```python
from build123d import *

# Parameters (mm, degrees)
F0_R     = 8
F1_DEPTH = 1
F3_DEPTH = 7
F4_R     = 8
F5_DEPTH = 1
F6_R     = 2.5
F7_DEPTH = 9


with BuildPart() as f1:
    # F0 (on Top) → F1 (new body)
    with BuildSketch(Plane.XY):
        Circle(F0_R)
    extrude(amount=F1_DEPTH)

    # F2 (on face) → F3 (join)
    with BuildSketch(Plane.XY.offset(1)):
        with BuildLine():
            Line((3.2969840058, 5.4029047423), (2.5065493984, 5.8119440209))
            ThreePointArc((2.5065493984, 5.8119440209), (1.8388116131, 5.5402736363), (1.4660287385, 6.1572918501))
            Line((1.4660287385, 6.1572918501), (0.587880666, 6.3020535948))
            ThreePointArc((0.587880666, 6.3020535948), (0.0367750598, 5.8373373817), (-0.5084316362, 6.3089603312))
            Line((-0.5084316362, 6.3089603312), (-1.3883339221, 6.1752742538))
            ThreePointArc((-1.3883339221, 6.1752742538), (-1.3836134942, 6.133709972), (-1.3820370329, 6.0919082168))
            ThreePointArc((-1.3820370329, 6.0919082168), (-1.8091754115, 5.5518374754), (-2.4331231799, 5.843063818))
            Line((-2.4331231799, 5.843063818), (-3.2286487127, 5.4440160432))
            ThreePointArc((-3.2286487127, 5.4440160432), (-3.1846641182, 5.3230332658), (-3.1697348597, 5.1951716444))
            ThreePointArc((-3.1697348597, 5.1951716444), (-3.5139617494, 4.6817520343), (-4.1196436741, 4.8052075072))
            Line((-4.1196436741, 4.8052075072), (-4.7529208721, 4.1798596116))
            ThreePointArc((-4.7529208721, 4.1798596116), (-4.6344100765, 4.0006685847), (-4.5928296865, 3.7898954745))
            ThreePointArc((-4.5928296865, 3.7898954745), (-4.859335021, 3.3157690905), (-5.4029047423, 3.2969840058))
            Line((-5.4029047423, 3.2969840058), (-5.8119440209, 2.5065493984))
            ThreePointArc((-5.8119440209, 2.5065493984), (-5.5928926927, 2.3021325953), (-5.5120190767, 2.0136379298))
            ThreePointArc((-5.5120190767, 2.0136379298), (-5.707906552, 1.590479337), (-6.1572918501, 1.4660287385))
            Line((-6.1572918501, 1.4660287385), (-6.3020535948, 0.587880666))
            ThreePointArc((-6.3020535948, 0.587880666), (-5.9691677754, 0.3993839994), (-5.8373263682, 0.0402714747))
            ThreePointArc((-5.8373263682, 0.0402714747), (-5.9714385265, -0.3214997579), (-6.3089603312, -0.5084316362))
            Line((-6.3089603312, -0.5084316362), (-6.1752742538, -1.3883339221))
            ThreePointArc((-6.1752742538, -1.3883339221), (-5.7301369842, -1.5161491913), (-5.5369082168, -1.9370370329))
            ThreePointArc((-5.5369082168, -1.9370370329), (-5.6196087137, -2.228512897), (-5.843063818, -2.4331231799))
            Line((-5.843063818, -2.4331231799), (-5.4440160432, -3.2286487127))
            ThreePointArc((-5.4440160432, -3.2286487127), (-4.9036957803, -3.2524353565), (-4.6401716444, -3.7247348597))
            ThreePointArc((-4.6401716444, -3.7247348597), (-4.683090061, -3.938738252), (-4.8052075072, -4.1196436741))
            Line((-4.8052075072, -4.1196436741), (-4.1798596116, -4.7529208721))
            ThreePointArc((-4.1798596116, -4.7529208721), (-3.5758920821, -4.6357481031), (-3.2348954745, -5.1478296865))
            ThreePointArc((-3.2348954745, -5.1478296865), (-3.2506409589, -5.2790911335), (-3.2969840058, -5.4029047423))
            Line((-3.2969840058, -5.4029047423), (-2.5065493984, -5.8119440209))
            ThreePointArc((-2.5065493984, -5.8119440209), (-1.8823764829, -5.5277645611), (-1.4586379298, -6.0670190767))
            ThreePointArc((-1.4586379298, -6.0670190767), (-1.4604887179, -6.1123064857), (-1.4660287385, -6.1572918501))
            Line((-1.4660287385, -6.1572918501), (-0.587880666, -6.3020535948))
            ThreePointArc((-0.587880666, -6.3020535948), (-0.0367750598, -5.8373373817), (0.5084316362, -6.3089603312))
            Line((0.5084316362, -6.3089603312), (1.3883339221, -6.1752742538))
            ThreePointArc((1.3883339221, -6.1752742538), (1.7688612926, -5.5630018732), (2.4331231799, -5.843063818))
            Line((2.4331231799, -5.843063818), (3.2286487127, -5.4440160432))
            ThreePointArc((3.2286487127, -5.4440160432), (3.4013491773, -4.7441209815), (4.1196436741, -4.8052075072))
            Line((4.1196436741, -4.8052075072), (4.7529208721, -4.1798596116))
            ThreePointArc((4.7529208721, -4.1798596116), (4.7008893059, -3.460852474), (5.4029047423, -3.2969840058))
            Line((5.4029047423, -3.2969840058), (5.8119440209, -2.5065493984))
            ThreePointArc((5.8119440209, -2.5065493984), (5.5402736363, -1.8388116131), (6.1572918501, -1.4660287385))
            Line((6.1572918501, -1.4660287385), (6.3020535948, -0.587880666))
            ThreePointArc((6.3020535948, -0.587880666), (5.8373373817, -0.0367750598), (6.3089603312, 0.5084316362))
            Line((6.3089603312, 0.5084316362), (6.1752742538, 1.3883339221))
            ThreePointArc((6.1752742538, 1.3883339221), (5.5630018732, 1.7688612926), (5.843063818, 2.4331231799))
            Line((5.843063818, 2.4331231799), (5.4440160432, 3.2286487127))
            ThreePointArc((5.4440160432, 3.2286487127), (4.7441209815, 3.4013491773), (4.8052075072, 4.1196436741))
            Line((4.8052075072, 4.1196436741), (4.1798596116, 4.7529208721))
            ThreePointArc((4.1798596116, 4.7529208721), (3.460852474, 4.7008893059), (3.2969840058, 5.4029047423))
        make_face()
    extrude(amount=F3_DEPTH)

    # F4 (on face) → F5 (join)
    with BuildSketch(Plane.XY.offset(8)):
        Circle(F4_R)
    extrude(amount=F5_DEPTH)

    # F6 (on face) → F7 (cut)
    with BuildSketch(Plane.XY.offset(9)):
        Circle(F6_R)
    extrude(amount=-F7_DEPTH, mode=Mode.SUBTRACT)


solid = f1.part
```
Model file for the job. Use its own axes, mm. A direction names the side the tool comes from. Coordinates: 2 decimals unless noted, no trailing zeros. Write each loop counter-clockwise with the first axis right and the second up, starting at its lowest first coordinate (ties: lowest second). Pieces come first, ordered by that corner, then holes. Notation, with made-up numbers: (-9.75, 39.5) - (48.25, 39.5) arc R19 cw to (48.25, 65.5) - close; hole circle Ø6 at (85.5, -14.75). An arc over 180 degrees is marked (long way). Use a Markdown table: item, result. Add a question column.
Item 1: Band-saw the part on A-A, the plane x = 0. Write the cut outline in (y, z), and give its area (3 significant figures).
Item 2: Two-plate mould, pull along Y, no slides. Class faces 1 (the face through (0.048, 5.837, 4.451)), 2 (the face through (-6.243, -0.942, 4.451)), 3 (the face through (5.837, -0.048, 4.451)): pulls with the +Y half, pulls with the -Y half, needs draft (parallel to the pull), parting line crosses it, or undercut.
Item 3: Drill centre lines: line 1 along Z through (x, y) = (2, 6.5); line 2 along Y through (x, z) = (0, 5.5); line 3 along X through (y, z) = (1.5, 0.75). Where is each one in solid material? Low to high.
Item 4: 3-axis set-ups, long thin cutter, end or side, ignore diameter. For faces 4 (the face through (-1.73, -7.81, 8.49)), 5 (the face through (-6.23, 1.03, 4.45)), 6 (the face through (3.47, 4.694, 4.451)), 7 (the face through (1.03, 6.23, 4.45)), 8 (the face through (0.942, -6.243, 4.451)): which of +Z, -Z, +X, -X, +Y, -Y reach the whole face in a straight line?
Item 5: Band-saw the part on B-B, the plane z = 8.5. Write the cut outline in (x, y), and give its area (3 significant figures).
Item 6: Drop flat-ended pins along their axis: pin 1 (4.5 mm diameter, centred on x = 0, y = 0, fed in from -Z); pin 2 (2 mm diameter, centred on x = 1, z = 2.5, fed in from +Y). Give the stop position or say it passes through.
A:
| question | item | result |
|---|---|---|
| 1 | outline | (-8, 0) - (-2.5, 0) - (-2.5, 9) - (-8, 9) - (-8, 8) - (-5.84, 8) - (-5.84, 1) - (-8, 1) - close; (2.5, 0) - (8, 0) - (8, 1) - (5.84, 1) - (5.84, 8) - (8, 8) - (8, 9) - (2.5, 9) - close |
| 1 | area | 68.7 mm² |
| 2 | face 1 | pulls with the +Y half |
| 2 | face 2 | pulls with the -Y half |
| 2 | face 3 | undercut |
| 3 | line 1 | z = 0 to 1, 8 to 9 |
| 3 | line 2 | y = -5.84 to -2.5, 2.5 to 5.84 |
| 3 | line 3 | x = -7.86 to -2, 2 to 7.86 |
| 4 | face 4 | +Z, -Z |
| 4 | face 5 | -X, +Y |
| 4 | face 6 | none |
| 4 | face 7 | +X, +Y |
| 4 | face 8 | +X, -Y |
| 5 | outline | circle Ø16 at (0, 0); hole circle Ø5 at (0, 0) |
| 5 | area | 181 mm² |
| 6 | pin 1 | passes through |
| 6 | pin 2 | stops at y = 6.3 |
